from build123d import *

# Parameters (mm, degrees)
SKETCH1_R           = 3.175
BOSS_EXTRUDE1_DEPTH = 10


with BuildPart() as part:
    # Sketch1 → Boss-Extrude1 (new body)
    with BuildSketch(Plane.XY):
        with BuildLine():
            Line((-47.46444948, 0), (-47.46444948, 19.93))
            ThreePointArc((-47.46444948, 19.93), (-44.535517292, 27.001067812), (-37.46444948, 29.93))
            Line((-37.46444948, 29.93), (-32.278753178, 29.93))
            Line((-32.278753178, 29.93), (-29.769076862, 24.828075765))
            Line((-29.769076862, 24.828075765), (-27.259400546, 19.72615153))
            Line((-27.259400546, 19.72615153), (-29.195289257, 18.773872777))
            ThreePointArc((-29.195289257, 18.773872777), (-31.233008862, 16.929762135), (-31.988313386, 14.287308668))
            Line((-31.988313386, 14.287308668), (-31.988313386, 0))
            Line((-31.988313386, 0), (-47.46444948, 0))
        make_face()
        with Locations((-39.726381433, 19.93)):
            Circle(SKETCH1_R, mode=Mode.SUBTRACT)
    extrude(amount=BOSS_EXTRUDE1_DEPTH)


solid = part.part
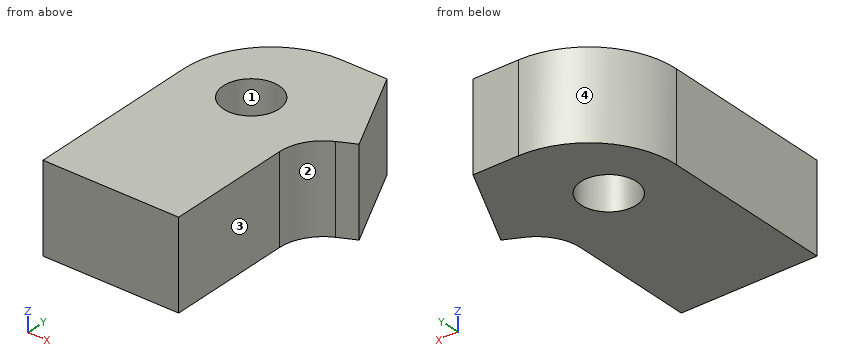
For this review, take the finished solid that the model builds, in its own axes (mm). Face numbers are marked on the shaded views. Coordinates: 2 decimals unless noted, no trailing zeros. Write each loop counter-clockwise with the first axis right and the second up, starting at its lowest first coordinate (ties: lowest second). Pieces come first, ordered by that corner, then holes. Notation, with made-up numbers: (40.5, -1) -> (59.5, -1) arc R28 cw to (59.5, 32) -> close; hole circle Ø2 at (35, -1.5). An arc over 180 degrees is marked (long way). Write each question's results on one line, items separated by ' | '. Start each with the question number.
1) Insertion check: pin 1 (8 mm diameter, centred on x = -42, y = 10, fed in from -Z); pin 2 (2 mm diameter, centred on x = -45, z = 4.5, fed in from +Y); pin 3 (3 mm diameter, centred on x = -40, z = 3.5, fed in from +Y). Each pin has a flat end and moves straight along its axis. Give the tip position at first contact, or say it passes through.
2) Wall thickness on L1, parallel to X at y = 9.25, z = 4.5; L2, parallel to X at y = 19.25, z = 6.5; L3, parallel to Y at x = -37.75, z = 2: over which ranges is each line inside the solid? List them lowest first. Write a range as [from, to].
3) Consider section A-A (z = 8.5). Write out the cut boundary in (x, y) (3 decimals), plus the area to 3 significant figures.
4) The part is to be moulded in two halves that separate along Y. For the marked faces 1, 2, 3 and 4, say which applies: +Y half, -Y half, draft (parallel to the pull), parting line (faces both ways), or undercut.
5) Consider section B-B (x = -38.25). Write out the cut boundary in (y, z).
6) Consider section C-C (y = 21.75). Write out the cut boundary in (x, z), plus the area to 3 significant figures.
7) Consider section D-D (y = 2.25). Write out the cut boundary in (x, z).
Geometry says:
1) pin 1: z = 0 | pin 2: y = 27.5 | pin 3: y = 29.88
2) L1: [-47.46, -31.99] | L2: [-47.46, -42.83], [-36.63, -28.23] | L3: [0, 17.45], [22.41, 29.93]
3) outline: (-47.464, 0) -> (-31.988, 0) -> (-31.988, 14.287) arc R5 cw to (-29.195, 18.774) -> (-27.259, 19.726) -> (-32.279, 29.93) -> (-37.464, 29.93) arc R10 ccw to (-47.464, 19.93) -> close; hole circle Ø6.35 at (-39.726, 19.93) | area: 440 mm^2
4) face 1: undercut | face 2: -Y half | face 3: draft | face 4: +Y half
5) outline: (0, 0) -> (17.12, 0) -> (17.12, 10) -> (0, 10) -> close; (22.74, 0) -> (29.9, 0) -> (29.9, 10) -> (22.74, 10) -> close
6) outline: (-47.3, 0) -> (-42.33, 0) -> (-42.33, 10) -> (-47.3, 10) -> close; (-37.12, 0) -> (-28.25, 0) -> (-28.25, 10) -> (-37.12, 10) -> close | area: 138 mm^2
7) outline: (-47.46, 0) -> (-31.99, 0) -> (-31.99, 10) -> (-47.46, 10) -> close
